from build123d import *

# Parameters (mm, degrees)
F0_W     = 1.902476
F0_H     = 41.352222
F1_DEPTH = 50.8
F2_T     = -101.6
F3_W     = 169.909547
F3_H     = 62.310902
F4_DEPTH = 25.4


with BuildPart() as f1:
    # F0 (on Top) → F1 (new body)
    with BuildSketch(Plane.XY):
        with Locations((-132.789068, -12.408881)):
            Rectangle(F0_W, F0_H)
    extrude(amount=F1_DEPTH)

    # F2
    f2_openings = [f1.faces().sort_by_distance(p)[0] for p in [
        (-131.83783, -12.408881, 25.4),
    ]]
    offset(amount=F2_T, openings=f2_openings)

    # F3 (on face) → F4 (join)
    with BuildSketch(Plane.XZ.offset(33.084992)):
        with Locations((-89.321027, -8.516186)):
            Rectangle(F3_W, F3_H)
    extrude(amount=F4_DEPTH)


solid = f1.part
The model under review builds one solid part; all positions refer to its coordinate system, in mm. A direction names the side the tool comes from. Round coordinates to 2 decimals unless told otherwise and drop trailing zeros. Order: outer loops, then holes, each group sorted by start corner. A loop starts at its lowest first (then second) coordinate and runs counter-clockwise, first axis right, second up. Notation, with made-up numbers: (0, -8) -> (31, -8) arc R24 cw to (31, 30) -> close; hole circle Ø9 at (6, 9.25). An arc over 180 degrees is marked (long way). Use CSV: the item, a comma, the result in double quotes. Start each with the question number.
(1) Consider section A-A on z = 9.5. Write out the cut boundary in (x, y) (3 decimals), and give its area (3 significant figures).
(2) Wall thickness on probe 1 along Y at (x, z) = (-131, 19) (3 decimals); probe 2 along Z at (x, y) = (-132, -38); probe 3 along X at (y, z) = (-27, 8): over which ranges is each line inside the solid? List them lowest first. Write a range as from..to.
(3) Consider section C-C on y = -41.5. Write out the cut boundary in (x, z).
(4) Tool access review of faces 1 (the face through (-174.276, -46, -9)), 2 (the face through (-131.838, -13, 25)), 3 (the face through (-133.74, -13, 25)): name each direction out of +Z, -Z, +X, -X, +Y, -Y from which nothing blocks a thin tool from reaching the whole face with its end or side.
(5) Insertion check: pin 1 (20.5 mm diameter, centred on y = -2, z = 30, fed in from +X); pin 2 (1 mm diameter, centred on x = -102.5, z = 0, fed in from +Y) (3 decimals); pin 3 (1 mm diameter, centred on x = -132.5, z = 32.5, fed in from -Y) (3 decimals); pin 4 (12 mm diameter, centred on x = -53, z = 32.5, fed in from +Y). Each pin has a flat end and moves straight along its axis. Give the tip position at first contact, or say it passes through.
(6) Consider section B-B on x = -29.5. Write out the cut boundary in (y, z) (3 decimals), and give its area (3 significant figures).
Responses:
1,outline,"(-174.276, -58.485) -> (-4.366, -58.485) -> (-4.366, -33.085) -> (-131.838, -33.085) -> (-131.838, 8.267) -> (-133.74, 8.267) -> (-133.74, -33.085) -> (-174.276, -33.085) -> close"
1,area,"4,390 mm²"
2,probe 1,"-58.485..-33.085"
2,probe 2,"-39.67..22.64"
2,probe 3,"-133.74..-131.84"
3,outline,"(-174.28, -39.67) -> (-4.37, -39.67) -> (-4.37, 22.64) -> (-174.28, 22.64) -> close"
4,face 1,"+Z, -Z, -X, +Y, -Y"
4,face 2,"+Z, -Z, +X, +Y"
4,face 3,"+Z, -Z, -X, +Y"
5,pin 1,"x = -131.84"
5,pin 2,"y = -33.085"
5,pin 3,"y = -33.085"
5,pin 4,"through"
6,outline,"(-58.485, -39.672) -> (-33.085, -39.672) -> (-33.085, 22.639) -> (-58.485, 22.639) -> close"
6,area,"1,580 mm²"
